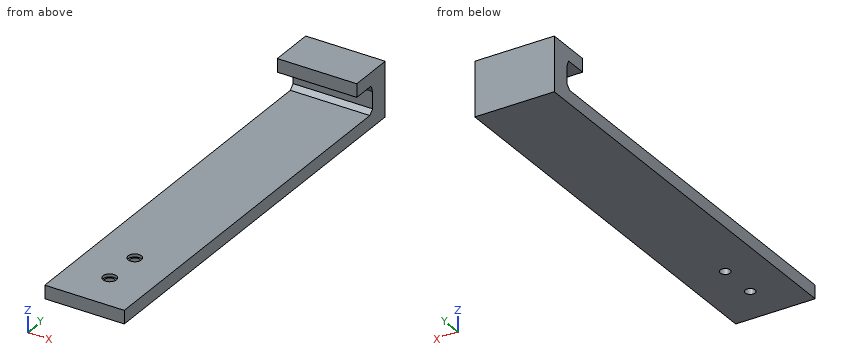
from build123d import *

# Parameters (mm, degrees)
F1_DEPTH = 25.4
F2_DEPTH = 112.776
F3_R     = 1.5875
F4_DEPTH = 25.4
F5_R     = 2.12725
F5_R_2   = 1.5875
F6_DEPTH = 0.9525


with BuildPart() as f1:
    # F0 (on Right) → F1 (new body)
    with BuildSketch(Plane.YZ):
        Polygon((0, 4.2545), (0, 0), (12.7, 0), (19.05, 0), (19.05, 4.2545), (19.05, 17.399), (12.7, 17.399), (4.699, 17.399), (4.699, 13.1445), (11.8730319638, 13.1445), (12.7, 11.0233025625), (12.7, 5.6484807283), (11.281458661, 4.2545), align=None)
    extrude(amount=F1_DEPTH)

    # F2 (add): a face of the model
    f2_faces = [f1.faces().sort_by_distance(p)[0] for p in [
        (12.7, 0, 2.12725),
    ]]
    extrude(f2_faces, amount=F2_DEPTH)

    # F3 (on face) → F4 (cut)
    with BuildSketch(Plane(origin=(0, 0, 0), x_dir=(1, 0, 0), z_dir=(0, 0, -1))):
        with Locations((12.7, 100.076)):
            Circle(F3_R)
        with Locations((12.7, 87.376)):
            Circle(F3_R)
    extrude(amount=-F4_DEPTH, mode=Mode.SUBTRACT)

    # F5 (on face) → F6 (cut)
    with BuildSketch(Plane.XY.offset(4.2545)):
        with Locations((12.7, -87.376)):
            Circle(F5_R)
        with Locations((12.7, -87.376)):
            Circle(F5_R_2, mode=Mode.SUBTRACT)
        with Locations((12.7, -100.076)):
            Circle(F5_R)
        with Locations((12.7, -100.076)):
            Circle(F5_R_2, mode=Mode.SUBTRACT)
    extrude(amount=-F6_DEPTH, mode=Mode.SUBTRACT)


solid = f1.part
Verification items for the finished model (mm, model axes). Give positions to 0.01 mm unless a question says otherwise; leave off trailing zeros. Write each loop counter-clockwise with the first axis right and the second up, starting at its lowest first coordinate (ties: lowest second). Pieces come first, ordered by that corner, then holes. Notation, with made-up numbers: (43, 85) -> (83, 85) arc R22 cw to (83, 123) -> close; hole circle Ø3 at (37, 6.5). An arc over 180 degrees is marked (long way). Use CSV: the item, a comma, the result in double quotes.
(1) Material ranges on L1, parallel to Y at x = 12.7, z = 3.85; L2, parallel to X at y = -87.5, z = 2; L3, parallel to Z at x = 21, y = 4, recorded low to high.
Derived:
L1,"y = -112.78 to -102.2, -97.95 to -89.5, -85.25 to 19.05"
L2,"x = 0 to 11.12, 14.28 to 25.4"
L3,"z = 0 to 4.25"
(2) Go/stop test with flat-tipped pins: pin 1 (4 mm diameter, centred on x = 10, y = -58.5, fed in from -Z); pin 2 (10 mm diameter, centred on x = 10, y = -80, fed in from +Z); pin 3 (3 mm diameter, centred on x = 21.5, z = 6, fed in from -Y); pin 4 (1.6 mm diameter, centred on x = 13.5, z = 7, fed in from -Y). Record where each tip stops, or that it passes through.
Derived:
pin 1,"stops at z = 0"
pin 2,"stops at z = 4.25"
pin 3,"stops at y = 11.53"
pin 4,"stops at y = 12.7"
(3) Sectioned sample at D-D (y = -35). Record the cut outline in (x, z), plus the area to 3 significant figures.
Derived:
outline,"(0, 0) -> (25.4, 0) -> (25.4, 4.25) -> (0, 4.25) -> close"
area,"108 mm^2"
(4) Sectioned sample at B-B (x = 19). Record the cut outline in (y, z).
Derived:
outline,"(-112.78, 0) -> (19.05, 0) -> (19.05, 17.4) -> (4.7, 17.4) -> (4.7, 13.14) -> (11.87, 13.14) -> (12.7, 11.02) -> (12.7, 5.65) -> (11.28, 4.25) -> (-112.78, 4.25) -> close"
(5) Sectioned sample at A-A (x = 12.7). Record the cut outline in (y, z), plus the area to 3 significant figures.
Derived:
outline,"(-112.78, 0) -> (-101.66, 0) -> (-101.66, 3.3) -> (-102.2, 3.3) -> (-102.2, 4.25) -> (-112.78, 4.25) -> close; (-98.49, 0) -> (-88.96, 0) -> (-88.96, 3.3) -> (-89.5, 3.3) -> (-89.5, 4.25) -> (-97.95, 4.25) -> (-97.95, 3.3) -> (-98.49, 3.3) -> close; (-85.79, 0) -> (19.05, 0) -> (19.05, 17.4) -> (4.7, 17.4) -> (4.7, 13.14) -> (11.87, 13.14) -> (12.7, 11.02) -> (12.7, 5.65) -> (11.28, 4.25) -> (-85.25, 4.25) -> (-85.25, 3.3) -> (-85.79, 3.3) -> close"
area,"651 mm^2"
(6) Sectioned sample at C-C (z = 8.75). Record the cut outline in (x, y).
Derived:
outline,"(0, 12.7) -> (25.4, 12.7) -> (25.4, 19.05) -> (0, 19.05) -> close"
